Autodesk Inventor part; units mm, degrees
ref_plane "YZ Plane" through (0, 0, 0) normal (1, 0, 0) x (0, 1, 0)
ref_plane "XZ Plane" through (0, 0, 0) normal (0, 1, 0) x (-1, 0, 0)
ref_plane "XY Plane" through (0, 0, 0) normal (0, 0, 1) x (1, 0, 0)
sketch "Sketch1" plane through (0, 0, 0) normal (0, 1, 0) x (-1, 0, 0)
  line L0 (0, 0) -> (120, 0)
  line L1 (120, 0) -> (120, -150)
  line L2 (120, -150) -> (0, -150)
  line L3 (0, -150) -> (0, 0)
  dimension "d0" = 120
  dimension "d1" = 150
extrude "Extrusion1" add sketch "Sketch1" along normal blind 90
shell "Shell1" thickness 8 removed faces 1 at (-80, 90, -100)
sketch "Sketch2" plane through (-120, 0, 0) normal (0, 0, 1) x (1, 0, 0)
  line L0 (120, 0) -> (0, 0)
  line L1 (0, 0) -> (0, 90)
  line L2 (86.681, 70.681) -> (33.319, 70.681)
  line L3 (33.319, 70.681) -> (33.319, 19.319)
  line L4 (33.319, 19.319) -> (86.681, 19.319)
  line L5 (86.681, 19.319) -> (86.681, 70.681)
  line L6 (86.681, 70.681) -> (33.319, 19.319) construction
  line L7 (33.319, 70.681) -> (86.681, 19.319) construction
  dimension "d5" = 53.362
  dimension "d6" = 51.362
extrude "Extrusion2" cut sketch "Sketch2" against normal blind 80
properties part number "case"
Could you check a few things on this model? Use its own coordinates, in mm. A direction names the side the tool comes from. Coordinates: 2 decimals unless noted, no trailing zeros. Order: outer loops, then holes, each group sorted by start corner. A loop starts at its lowest first (then second) coordinate and runs counter-clockwise, first axis right, second up. Notation, with made-up numbers: M 23,83 L 32,83 A12 ccw 32,106 Z; hole C -38.5,-15 d9. An arc over 180 degrees is marked long. Use a Markdown table: item, result. Add a question column.
Q1. Which directions (+Z, -Z, +X, -X, +Y, -Y) give clear straight access to the entire face, cutting with the end or side of a thin tool? Please do faces 4 (the flat face through (-59, 8, -74)), 5 (the flat face through (-60, 19.319, -4)), 6 (the flat face through (-120, 44, -74)).
Q2. We'd pull the mould along X, two halves only. Please class faces 1 (the flat face through (0, 44, -76)), 2 (the flat face through (-6, 90, -69)), 3 (the flat face through (-33.319, 45, -4)): pulls with the +X half, pulls with the -X half, needs draft (parallel to the pull), parting line crosses it, or undercut.
Q3. I want a section at D-D on x = -104. List the corners of the cut face in (y, z) for me.
Q4. I want a section at A-A on y = 76.5. List the corners of the cut face in (x, z) for me.
Q5. I want a section at C-C on x = -36.5. List the corners of the cut face in (y, z) for me, then the cut area to 3 significant figures.
Q6. I want a section at B-B on z = -14.5. List the corners of the cut face in (x, y) for me.
Q7. If I drill on L1, parallel to Z at x = -20.5, y = 40; L2, parallel to X at y = 42.5, z = -127.5; L3, parallel to Y at x = -94, z = -113, over which ranges is the centre line in solid material (lowest first)?
Q8. I'm going to push a flat-ended pin straight in: pin 1 (3 mm diameter, centred on x = -82.5, y = 51.5, fed in from +Z). Where does the tip first touch, or does it pass through?
Checked values:
| question | item | result |
|---|---|---|
| 1 | face 4 | +Y |
| 1 | face 5 | +Z |
| 1 | face 6 | +Z, -Z, -X, +Y, -Y |
| 2 | face 1 | pulls with the +X half |
| 2 | face 2 | needs draft |
| 2 | face 3 | undercut |
| 3 | outline | M 0,-150 L 90,-150 L 90,-142 L 8,-142 L 8,-8 L 90,-8 L 90,0 L 0,0 Z |
| 4 | outline | M -120,-150 L 0,-150 L 0,0 L -120,0 Z; hole M -112,-142 L -8,-142 L -8,-8 L -112,-8 Z |
| 5 | outline | M 0,-150 L 90,-150 L 90,-142 L 8,-142 L 8,-8 L 19.32,-8 L 19.32,0 L 0,0 Z; M 70.68,-8 L 90,-8 L 90,0 L 70.68,0 Z |
| 5 | area | 2,100 mm² |
| 6 | outline | M -120,0 L 0,0 L 0,90 L -8,90 L -8,8 L -112,8 L -112,90 L -120,90 Z |
| 7 | L1 | -150 to -142, -8 to 0 |
| 7 | L2 | -120 to -112, -8 to 0 |
| 7 | L3 | 0 to 8 |
| 8 | pin 1 | z = -142 |
